The listing builds one solid part. Answer for the finished solid, in the listing's coordinates (mm). A direction names the side the tool comes from. Coordinates: 2 decimals unless noted, no trailing zeros. Order: outer loops, then holes, each group sorted by start corner. A loop starts at its lowest first (then second) coordinate and runs counter-clockwise, first axis right, second up. Notation, with made-up numbers: (28.5, 54) -> (59.5, 54) arc R24 ccw to (59.5, 80) -> close; hole circle Ø6 at (88, 64). An arc over 180 degrees is marked (long way). Return JSON: item names as keys, results as strings.
Autodesk Fusion 360 part; units mm, degrees
sketch "草图1" plane through (0, 0, 0) normal (0, 0, 1) x (1, 0, 0)
  circle A0 centre (0, 0) radius 26.15 construction
  circle A1 centre (0, 0) radius 25.5 construction
  circle A2 centre (0, 0) radius 31
  line L0 (0, 0) -> (46, 0) construction
  line L1 (0, 0) -> (0, 44.4165) construction
  line L2 (0, 0) -> (38.8757, 16.1028) construction
  circle A3 centre (23.5589, 9.7584) radius 2.35
  circle A4 centre (9.7584, 23.5589) radius 2.35
  circle A5 centre (-9.7584, 23.5589) radius 2.35
  circle A6 centre (-23.5589, 9.7584) radius 2.35
  circle A7 centre (-23.5589, -9.7584) radius 2.35
  circle A8 centre (-9.7584, -23.5589) radius 2.35
  circle A9 centre (9.7584, -23.5589) radius 2.35
  circle A10 centre (23.5589, -9.7584) radius 2.35
  dimension "d1" = 52.3
  dimension "d2" = 51
  dimension "d3" = 62
  dimension "d4" = 22.5
  dimension "d5" = 4.7
  dimension "d8" = 0
  dimension "d9" = 0
  dimension "d11" = 360
ref_plane "工作平面1" through (0, 0, 50) normal (0, 0, 1) x (1, 0, 0)
sketch "草图2" plane through (0, 0, 50) normal (0, 0, 1) x (1, 0, 0)
  circle A0 centre (0, 0) radius 26.15
  circle A1 centre (0, 0) radius 19.8 construction
  line L0 (0, 0) -> (28.4429, 28.4429) construction
  line L1 (0, 0) -> (40.2244, 0) construction
  circle A2 centre (14.0007, 14.0007) radius 1.5
  circle A3 centre (-14.0007, 14.0007) radius 1.5
  circle A4 centre (-14.0007, -14.0007) radius 1.5
  circle A5 centre (14.0007, -14.0007) radius 1.5
  circle A6 centre (14.0007, 14.0007) radius 1.5
  circle A7 centre (-14.0007, 14.0007) radius 1.5
  circle A8 centre (-14.0007, -14.0007) radius 1.5
  circle A9 centre (14.0007, -14.0007) radius 1.5
  dimension "d13" = 52.3
  dimension "d14" = 39.6
  dimension "d15" = 45
  dimension "d16" = 3
  dimension "d18" = 360
  dimension "d19" = 3
loft "放样1" add profiles "草图1", "草图2" section 1 section 2
sketch "草图3" plane through (0, 0, 50) normal (0, 0, 1) x (-1, 0, 0)
  circle A0 centre (0, 0) radius 26.15
  line L0 (0, 0) -> (-33, 0) construction
  line L1 (0, 0) -> (0, -36) construction
  line L2 (0, 0) -> (-34.5137, -34.5137) construction
  circle A1 centre (0, 0) radius 19.8 construction
  circle A2 centre (-14.0007, -14.0007) radius 1.5
  circle A3 centre (14.0007, -14.0007) radius 1.5
  circle A4 centre (14.0007, 14.0007) radius 1.5
  circle A5 centre (-14.0007, 14.0007) radius 1.5
  dimension "d20" = 45
  dimension "d21" = 39.6
  dimension "d22" = 3
  dimension "d24" = 360
hole "孔1" at (14.0007, 14.0007, 50) at (-14.0007, 14.0007, 50) at (-14.0007, -14.0007, 50) at (14.0007, -14.0007, 50) direction (0, 0, -1) diameter 3 depth 10 tip angle 118
sketch "草图4" plane through (0, 0, 0) normal (0, 0, -1) x (1, 0, 0)
  circle A0 centre (0, 0) radius 31
  line L0 (0, 0) -> (47.5733, 0) construction
  line L1 (0, 0) -> (0, -48.4854) construction
  line L2 (0, 0) -> (51.3087, -21.2528) construction
  circle A1 centre (0, 0) radius 25.5 construction
  circle A2 centre (23.5589, -9.7584) radius 2.35
  circle A3 centre (23.5589, 9.7584) radius 2.35
  circle A4 centre (9.7584, 23.5589) radius 2.35
  circle A5 centre (-9.7584, 23.5589) radius 2.35
  circle A6 centre (-23.5589, 9.7584) radius 2.35
  circle A7 centre (-23.5589, -9.7584) radius 2.35
  circle A8 centre (-9.7584, -23.5589) radius 2.35
  circle A9 centre (9.7584, -23.5589) radius 2.35
  dimension "d28" = 22.5
  dimension "d29" = 51
  dimension "d30" = 4.7
  dimension "d32" = 360
hole "孔2" at (9.7584, -23.5589, 0) at (-9.7584, -23.5589, 0) at (-23.5589, -9.7584, 0) at (-23.5589, 9.7584, 0) at (-9.7584, 23.5589, 0) at (9.7584, 23.5589, 0) at (23.5589, 9.7584, 0) at (23.5589, -9.7584, 0) direction (0, 0, 1) diameter 4.7 depth 10 tip angle 180
hole "孔3" at (0, 0, 0) direction (0, 0, 1) diameter 30 end through all
1. The part is cut by section B-B on z = 3. Give the number of separate pieces and of enclosed holes in the cut face, and give its area (3 significant figures).
Answer block:
{"separate pieces": "1", "enclosed holes": "9", "area": "2,120 mm2"}
2. Determine the mould class of faces 1 (the face through (13.3, 7.3, 0)), 2 (the face through (14.575, 12.615, 44.93)), 3 (the face through (11.19, -25.42, 5.07)) for opening direction X: pulls with the +X half, pulls with the -X half, needs draft (parallel to the pull), parting line crosses it, or undercut.
Answer block:
{"face 1": "needs draft", "face 2": "undercut", "face 3": "undercut"}
3. Consider line 1 (Y direction, x = 0, z = 44); line 2 (Y direction, x = -2.5, z = 43); line 3 (X direction, y = 3.5, z = 47.5). Determine where each line is inside the solid, lowest interval first. Write a range as from..to.
Answer block:
{"line 1": "y = -26.73..-15, 15..26.73", "line 2": "y = -26.71..-14.79, 14.79..26.71", "line 3": "x = -26.16..-14.59, 14.59..26.16"}
4. The part is cut by section C-C on z = 41.5. Give the vertices of the cut face in (x, y).
Answer block:
{"outline": "circle Ø53.95 at (0, 0); hole circle Ø3 at (-14, -14); hole circle Ø3 at (-14, 14); hole circle Ø30 at (0, 0); hole circle Ø3 at (14, -14); hole circle Ø3 at (14, 14)"}
5. Each of these flat-tipped pins is pushed along its axis until it touches: pin 1 Ø2 at (x, y) = (10.5, -13.5) entering from -Z; pin 2 Ø1.4 at (x, y) = (9, 24.5) entering from -Z; pin 3 Ø12 at (y, z) = (1.5, 42.5) entering from -X; pin 4 Ø1.5 at (y, z) = (21, 39) entering from -X. Where does it stop, or does it pass through?
Answer block:
{"pin 1": "stops at z = 0", "pin 2": "stops at z = 10", "pin 3": "stops at x = -27.45", "pin 4": "stops at x = -18.19"}
6. The part is cut by section A-A on x = 0. Give the vertices of the cut face in (y, z), and give its area (3 significant figures).
Answer block:
{"outline": "(-31, 0) -> (-15, 0) -> (-15, 50) -> (-26.15, 50) -> close; (15, 0) -> (31, 0) -> (26.15, 50) -> (15, 50) -> close", "area": "1,360 mm2"}
7. For faces 4 (the face through (11, -11, 50)), 5 (the face through (-21.265, 9.249, 5.07)), determine the directions among +Z, -Z, +X, -X, +Y, -Y from which every point of the face is accessible in a straight line to the end or side of a thin tool.
Answer block:
{"face 4": "+Z, +X, -X, +Y, -Y", "face 5": "-Z"}
8. The part is cut by section D-D on z = 14. Give the vertices of the cut face in (x, y).
Answer block:
{"outline": "circle Ø59.28 at (0, 0); hole circle Ø30 at (0, 0)"}
